Source: CAD feature listing. Evaluate the final solid. Frame: model axes, mm. Give positions to 0.01 mm unless a question says otherwise; leave off trailing zeros. Order: outer loops, then holes, each group sorted by start corner. A loop starts at its lowest first (then second) coordinate and runs counter-clockwise, first axis right, second up.
```python
from build123d import *

# Parameters (mm, degrees)
BOSS_EXTRUDE1_DEPTH = 0.25


with BuildPart() as part:
    # Sketch1 → Boss-Extrude1 (new, symmetric)
    with BuildSketch(Plane(origin=(0, 0, 0), x_dir=(1, 0, 0), z_dir=(0, 1, 0))):
        with BuildLine():
            Line((1.977113733, 26.118743762), (1.977113733, 38.118743762))
            Line((1.977113733, 38.118743762), (-15.022886267, 38.118743762))
            Line((-15.022886267, 38.118743762), (-15.022886267, 19.393587035))
            Line((-15.022886267, 19.393587035), (-10.522886267, 19.393587035))
            Line((-10.522886267, 19.393587035), (-10.522886267, 28.893587035))
            Line((-10.522886267, 28.893587035), (-9.772886267, 28.893587035))
            ThreePointArc((-9.772886267, 28.893587035), (-8.022886267, 30.643587035), (-6.272886267, 28.893587035))
            Line((-6.272886267, 28.893587035), (-5.522886267, 28.893587035))
            Line((-5.522886267, 28.893587035), (-5.522886267, 23.718587035))
            ThreePointArc((-5.522886267, 23.718587035), (-4.358162581, 25.477926708), (-2.347886267, 26.118743762))
            Line((-2.347886267, 26.118743762), (1.977113733, 26.118743762))
        make_face()
    extrude(amount=BOSS_EXTRUDE1_DEPTH, both=True)


solid = part.part
```
1) Section query B-B, the plane y = 0.1. Return the cut outline in (x, z) (3 decimals), and give its area (3 significant figures).
Report:
outline: (-15.023, -38.119) - (1.977, -38.119) - (1.977, -26.119) - (-2.348, -26.119) arc R3.175 cw to (-5.523, -23.719) - (-5.523, -28.894) - (-6.273, -28.894) arc R1.75 cw to (-9.773, -28.894) - (-10.523, -28.894) - (-10.523, -19.394) - (-15.023, -19.394) - close
area: 217 mm2
2) Section query A-A, the plane z = -28.5. Return the cut outline in (x, y).
Report:
outline: (-15.02, -0.25) - (-10.52, -0.25) - (-10.52, 0.25) - (-15.02, 0.25) - close; (-5.52, -0.25) - (1.98, -0.25) - (1.98, 0.25) - (-5.52, 0.25) - close
3) Section query D-D, the plane z = -22.25. Return the cut outline in (x, y).
Report:
outline: (-15.02, -0.25) - (-10.52, -0.25) - (-10.52, 0.25) - (-15.02, 0.25) - close
4) Draft query along X for faces 1 (the flat face through (-7, 0.25, -31)), 2 (the cylindrical face through (-8.061, 0.004, -30.643)). Return one class per face: +X half, -X half, draft (parallel to the pull), parting line (faces both ways), or undercut.
Report:
face 1: draft
face 2: undercut
5) Material intervals for L1, parallel to X at y = 0, z = -26.25; L2, parallel to Z at x = 0.75, y = 0.05; L3, parallel to Z at x = -10, y = 0.2, sorted ascending.
Report:
L1: x = -15.02 to -10.52, -5.52 to 1.98
L2: z = -38.12 to -26.12
L3: z = -38.12 to -28.89
6) Section query C-C, the plane x = -1.75. Return the cut outline in (y, z).
Report:
outline: (-0.25, -38.12) - (0.25, -38.12) - (0.25, -26.12) - (-0.25, -26.12) - close
